from build123d import *

# Parameters (mm, degrees)
SKETCH1_R           = 1.4986
BOSS_EXTRUDE1_DEPTH = 2.3114


with BuildPart() as part:
    # Sketch1 → Boss-Extrude1 (new body)
    with BuildSketch(Plane(origin=(0, 0, 0), x_dir=(1, 0, 0), z_dir=(0, 1, 0))):
        with BuildLine():
            Line((-2.4511, -3.937), (-2.4511, 3.937))
            ThreePointArc((-2.4511, 3.937), (0, 6.3881), (2.4511, 3.937))
            Line((2.4511, 3.937), (2.4511, -3.937))
            ThreePointArc((2.4511, -3.937), (0, -6.3881), (-2.4511, -3.937))
        make_face()
        with Locations((0, 3.937)):
            Circle(SKETCH1_R, mode=Mode.SUBTRACT)
        with Locations((0, -3.937)):
            Circle(SKETCH1_R, mode=Mode.SUBTRACT)
        Circle(SKETCH1_R, mode=Mode.SUBTRACT)
    extrude(amount=BOSS_EXTRUDE1_DEPTH)


solid = part.part
CAD build for the part. Positions are in the model's coordinates, mm. Round coordinates to 2 decimals unless told otherwise and drop trailing zeros. Order: outer loops, then holes, each group sorted by start corner. A loop starts at its lowest first (then second) coordinate and runs counter-clockwise, first axis right, second up. Notation, with made-up numbers: (54, 33) - (73, 33) arc R33 cw to (73, 66) - close; hole circle Ø5 at (5.5, -38.5). An arc over 180 degrees is marked (long way). Return JSON: item names as keys, results as strings.
(1) Pull direction Z, two halves, no side cores. Call faces 1 (the face through (-0.32, 1.14, 5.4)), 2 (the face through (2.451, 1, 0)), 3 (the face through (1.43, 1.14, -0.45)), 4 (the face through (0.054, 1.14, 6.388)): +Z half, -Z half, draft (parallel to the pull), parting line (faces both ways), or undercut.
Answer key:
{"face 1": "undercut", "face 2": "draft", "face 3": "undercut", "face 4": "+Z half"}
(2) Cut at D-D (z = 5.25). Give the cut face in (x, y), then the cut area to 3 significant figures.
Answer key:
{"outline": "(-2.07, 0) - (-0.72, 0) - (-0.72, 2.31) - (-2.07, 2.31) - close; (0.72, 0) - (2.07, 0) - (2.07, 2.31) - (0.72, 2.31) - close", "area": "6.23 mm^2"}
(3) Cut at B-B (x = 0). Give the cut face in (y, z), then the cut area to 3 significant figures.
Answer key:
{"outline": "(0, -6.39) - (2.31, -6.39) - (2.31, -5.44) - (0, -5.44) - close; (0, -2.44) - (2.31, -2.44) - (2.31, -1.5) - (0, -1.5) - close; (0, 1.5) - (2.31, 1.5) - (2.31, 2.44) - (0, 2.44) - close; (0, 5.44) - (2.31, 5.44) - (2.31, 6.39) - (0, 6.39) - close", "area": "8.75 mm^2"}
(4) Cut at C-C (y = 1.8). Give the cut face in (x, z), then the cut area to 3 significant figures.
Answer key:
{"outline": "(-2.45, -3.94) arc R2.45 ccw to (2.45, -3.94) - (2.45, 3.94) arc R2.45 ccw to (-2.45, 3.94) - close; hole circle Ø3 at (0, -3.94); hole circle Ø3 at (0, 0); hole circle Ø3 at (0, 3.94)", "area": "36.3 mm^2"}
(5) Wall check: probe 1 along Z at (x, y) = (0, 1.4); probe 2 along X at (y, z) = (1.05, 0); probe 3 along Z at (x, y) = (-1.15, 0.8). Give the ranges that are in metal, low to high. Write a range as from..to.
Answer key:
{"probe 1": "z = -6.39..-5.44, -2.44..-1.5, 1.5..2.44, 5.44..6.39", "probe 2": "x = -2.45..-1.5, 1.5..2.45", "probe 3": "z = -6.1..-4.9, -2.98..-0.96, 0.96..2.98, 4.9..6.1"}
(6) Pin check, flat tip, straight feed: pin 1 Ø2 at (x, z) = (1.5, 4) entering from -Y. Stop position of the tip, or through.
Answer key:
{"pin 1": "stops at y = 0"}
(7) Cut at A-A (z = 0). Give the cut face in (x, y), then the cut area to 3 significant figures.
Answer key:
{"outline": "(-2.45, 0) - (-1.5, 0) - (-1.5, 2.31) - (-2.45, 2.31) - close; (1.5, 0) - (2.45, 0) - (2.45, 2.31) - (1.5, 2.31) - close", "area": "4.40 mm^2"}
